from build123d import *

# Parameters (mm, degrees)
BOSS_EXTRUDE1_DEPTH              = 19.05
F_1_8_0_125_DIAMETER_HOLE1_D     = 3.175
F_1_8_0_125_DIAMETER_HOLE1_DEPTH = 11.1252
F_1_8_0_125_DIAMETER_HOLE1_TIP   = 0.953866233
F_1_8_0_125_DIAMETER_HOLE2_D     = 3.175


with BuildPart() as part:
    # Sketch1 → Boss-Extrude1 (new body)
    with BuildSketch(Plane(origin=(0, 0, 0), x_dir=(1, 0, 0), z_dir=(0, 1, 0))):
        with BuildLine():
            Line((-257.175, 0), (257.175, 0))
            Line((257.175, 0), (257.175, -104.032493436))
            Line((257.175, -104.032493436), (199.670208733, -104.032493436))
            ThreePointArc((199.670208733, -104.032493436), (107.889594305, -43.469891278), (0, -22.225))
            Line((0, -22.225), (-127, -22.225))
            ThreePointArc((-127, -22.225), (-219.047625241, -60.352374759), (-257.175, -152.4))
            Line((-257.175, -152.4), (-276.225, -152.4))
            Line((-276.225, -152.4), (-276.225, -50.8))
            Line((-276.225, -50.8), (-257.175, -50.8))
            Line((-257.175, -50.8), (-257.175, 0))
        make_face()
    extrude(amount=BOSS_EXTRUDE1_DEPTH)

    # 1/8 (0.125) Diameter Hole1
    with Locations(Plane(origin=(0, 0, 0), x_dir=(-1, 0, 0), z_dir=(0, -1, 0))):
        with Locations((0, -11.1125), (225.425, -23.8125), (-225.425, -23.8125), (-225.425, -67.519993436), (257.175, -84.6005531)):
            Hole(F_1_8_0_125_DIAMETER_HOLE1_D / 2, depth=F_1_8_0_125_DIAMETER_HOLE1_DEPTH)
            with Locations((0, 0, -(F_1_8_0_125_DIAMETER_HOLE1_DEPTH + F_1_8_0_125_DIAMETER_HOLE1_TIP / 2))):  # 118° drill point
                Cone(0, F_1_8_0_125_DIAMETER_HOLE1_D / 2, F_1_8_0_125_DIAMETER_HOLE1_TIP, mode=Mode.SUBTRACT)

    # 1/8 (0.125) Diameter Hole2 (through all)
    with Locations(Plane(origin=(0, 19.05, 0), x_dir=(1, 0, 0), z_dir=(0, 1, 0))):
        with Locations((-246.552544448, -36.961239505), (-208.452544448, -36.961239505), (-246.552544448, -75.061239505), (-231.830017346, -51.683766607)):
            Hole(F_1_8_0_125_DIAMETER_HOLE2_D / 2)


solid = part.part
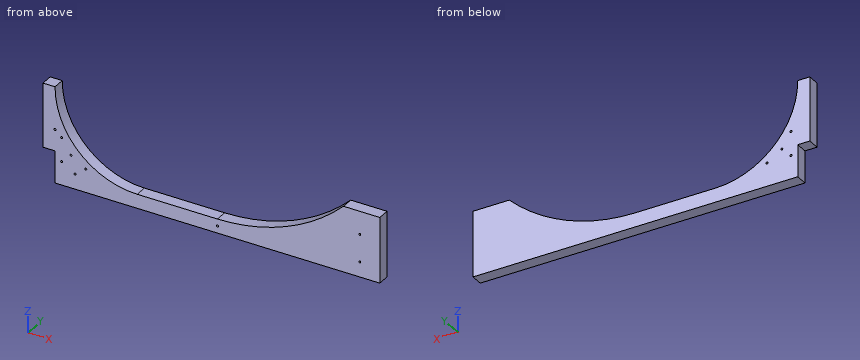
Input: part model. Units: mm. Frame: model coordinates. Coordinates: 2 decimals unless noted, no trailing zeros. Loops run counter-clockwise (first coordinate to the right, second up) from the corner with the lowest first, then second, coordinate; pieces in that order, holes last.
(1) Material intervals for probe 1 along X at (y, z) = (8.5, 76.5) (3 decimals); probe 2 along X at (y, z) = (12.75, 81) (3 decimals); probe 3 along Z at (x, y) = (-231, 2.5), sorted ascending.
(2) Section A-A on x = -77.5. Return the cut outline in (y, z) (3 decimals).
(3) First-contact query: pin 1 Ø4 at (x, z) = (225.42, 23.81) entering from -Y; pin 2 Ø2.5 at (x, z) = (-225.42, 23.81) entering from -Y; pin 3 Ø1.9 at (x, z) = (0, 11.11) entering from -Y; pin 4 Ø2 at (y, z) = (10.5, 128.5) entering from +X. Flat tips, straight axial feed; report the tip coordinate or a pass-through.
(4) Section C-C on z = 110.5. Return the cut outline in (x, y) (3 decimals), then the cut area to 3 significant figures.
(5) Section B-B on y = 4.5. Count the separate pieces of the cut face and the enclosed holes in it, then the cut area to 3 significant figures.
Data:
1. probe 1: x = -276.225 to -247.223, -245.882 to -232.758, 167.167 to 257.175
1. probe 2: x = -276.225 to -235.847, 173.197 to 257.175
1. probe 3: z = 0 to 50.33, 53.04 to 74.11
2. outline: (0, 0) - (19.05, 0) - (19.05, 22.225) - (0, 22.225) - close
3. pin 1: stops at y = 0
3. pin 2: stops at y = 11.32
3. pin 3: stops at y = 11.51
3. pin 4: stops at x = -254.77
4. outline: (-276.225, 0) - (-250.247, 0) - (-250.247, 19.05) - (-276.225, 19.05) - close
4. area: 495 mm2
5. separate pieces: 1
5. enclosed holes: 9
5. area: 26,700 mm2
